Here's how the part is built. I have some questions about the finished solid (model axes, mm). Round coordinates to 2 decimals unless told otherwise and drop trailing zeros. Write each loop counter-clockwise with the first axis right and the second up, starting at its lowest first coordinate (ties: lowest second). Pieces come first, ordered by that corner, then holes. Notation, with made-up numbers: (-19, 34) -> (-10, 34) arc R25 cw to (-10, 65) -> close; hole circle Ø10 at (25.5, 5). An arc over 180 degrees is marked (long way). Answer as CSV lines item,"result".
Autodesk Inventor part; units mm, degrees
ref_plane "YZ Plane" through (0, 0, 0) normal (1, 0, 0) x (0, 1, 0)
ref_plane "XZ Plane" through (0, 0, 0) normal (0, 1, 0) x (-1, 0, 0)
ref_plane "XY Plane" through (0, 0, 0) normal (0, 0, 1) x (1, 0, 0)
sketch "スケッチ1" plane through (0, 0, 0) normal (1, 0, 0) x (0, 1, 0)
  line L0 (-5, -5) -> (5, -5)
  line L1 (5, -5) -> (5, 5)
  line L2 (5, 5) -> (-5, 5)
  line L3 (-5, 5) -> (-5, -5)
  line L4 (-1, 5) -> (1, 5)
  line L5 (1, 5) -> (1, 3)
  line L6 (1, 3) -> (-1, 3)
  line L7 (-1, 3) -> (-1, 5)
  line L8 (3, -1) -> (5, -1)
  line L9 (5, -1) -> (5, 1)
  line L10 (5, 1) -> (3, 1)
  line L11 (3, 1) -> (3, -1)
  point P0 (0, 0)
  dimension "d0" = 5
  dimension "d1" = 5
  dimension "d2" = 5
  dimension "d3" = 5
  dimension "d4" = 2
  dimension "d5" = 1
  dimension "d6" = 2
  dimension "d7" = 1
  dimension "d8" = 2
  dimension "d9" = 2
extrude "押し出し1" add sketch "スケッチ1" along normal blind 250 contours L3 L2 L7 L6 L5 L1 L10 L11 L8 L0
properties part number "banper" material "PET プラスチック"
1. For pin 1 Ø0.6 at (x, z) = (68, 0.5) entering from +Y; pin 2 Ø0.6 at (x, y) = (79.5, 0) entering from +Z, each with a flat end and sliding along its axis, tell me the tip position at first contact or that it passes through.
Numbers:
pin 1,"stops at y = 3"
pin 2,"stops at z = 3"
2. If I drill on line 1 (Y direction, x = 224, z = 3.75); line 2 (Z direction, x = 112.5, y = -0.75), over which ranges is the centre line in solid material (lowest first)?
Numbers:
line 1,"y = -5 to -1, 1 to 5"
line 2,"z = -5 to 3"
3. Suppose I cut it at A-A on x = 183. Please give me the cut outline in (y, z).
Numbers:
outline,"(-5, -5) -> (5, -5) -> (5, -1) -> (3, -1) -> (3, 1) -> (5, 1) -> (5, 5) -> (1, 5) -> (1, 3) -> (-1, 3) -> (-1, 5) -> (-5, 5) -> close"
